Verification items for this drawing (mm, ordinates from the low corner). A direction names the side the tool comes from. Round coordinates to 2 decimals unless told otherwise and drop trailing zeros. Loops run counter-clockwise (first coordinate to the right, second up) from the corner with the lowest first, then second, coordinate; pieces in that order, holes last. Notation, with made-up numbers: M -3.75,-0.5 L 14.25,-0.5 A16 ccw 14.25,22.5 Z; hole C 2.5,68.5 d3. An arc over 180 degrees is marked long. Answer as CSV lines item,"result".
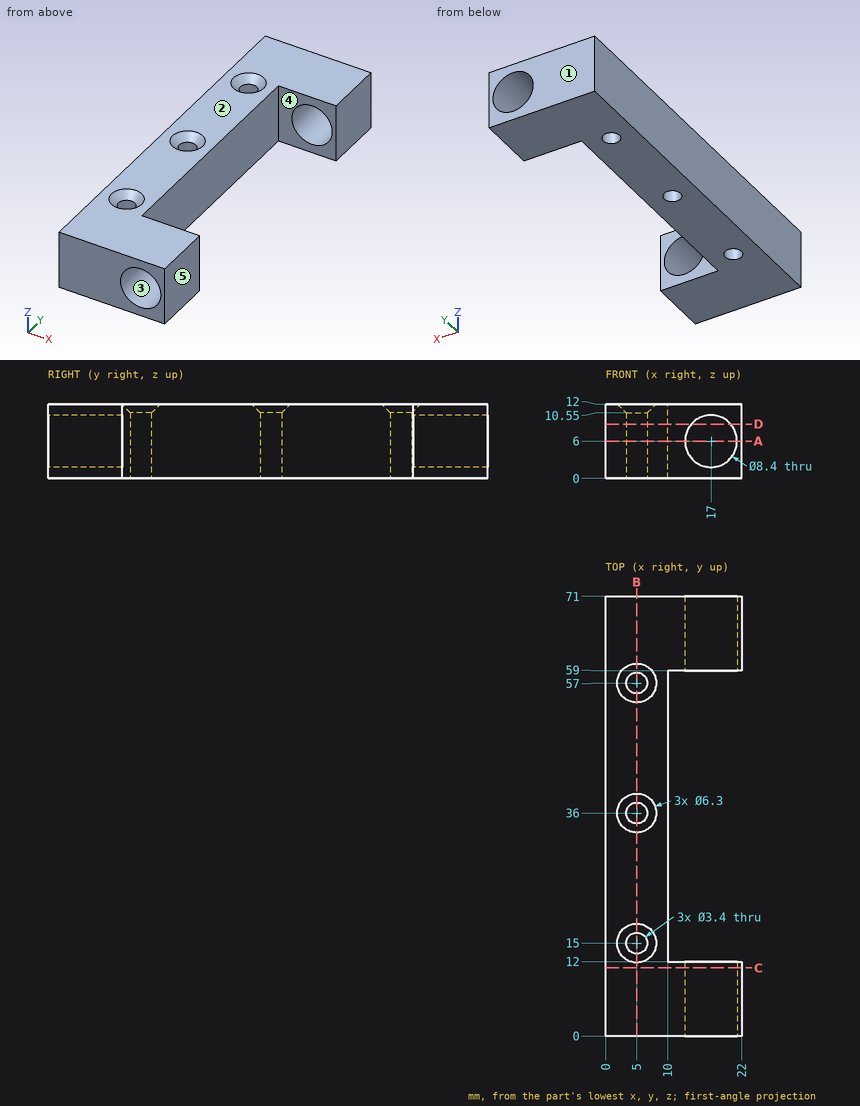
1) Section check C-C (y = 11). Record the cut outline in (x, z), plus the area to 3 significant figures.
Here are the results:
outline,"M 0,0 L 22,0 L 22,12 L 0,12 Z; hole C 17,6 d8.4"
area,"209 mm^2"
2) Section check D-D (z = 8.75). Record the cut outline in (x, y), plus the area to 3 significant figures.
Here are the results:
outline,"M 0,0 L 13.83,0 L 13.83,12 L 10,12 L 10,59 L 13.83,59 L 13.83,71 L 0,71 Z; M 20.17,0 L 22,0 L 22,12 L 20.17,12 Z; M 20.17,59 L 22,59 L 22,71 L 20.17,71 Z; hole C 5,15 d3.4; hole C 5,36 d3.4; hole C 5,57 d3.4"
area,"818 mm^2"
3) Draft check along Z on the marked faces 1, 2 and 3. Enter one of: +Z half, -Z half, draft (parallel to the pull), parting line (faces both ways), or undercut.
Here are the results:
face 1,"draft"
face 2,"+Z half"
face 3,"undercut"
4) Section check B-B (x = 5). Record the cut outline in (y, z), plus the area to 3 significant figures.
Here are the results:
outline,"M 0,0 L 13.3,0 L 13.3,10.55 L 11.85,12 L 0,12 Z; M 16.7,0 L 34.3,0 L 34.3,10.55 L 32.85,12 L 18.15,12 L 16.7,10.55 Z; M 37.7,0 L 55.3,0 L 55.3,10.55 L 53.85,12 L 39.15,12 L 37.7,10.55 Z; M 58.7,0 L 71,0 L 71,12 L 60.15,12 L 58.7,10.55 Z"
area,"723 mm^2"
5) Section check A-A (z = 6). Record the cut outline in (x, y).
Here are the results:
outline,"M 0,0 L 12.8,0 L 12.8,12 L 10,12 L 10,59 L 12.8,59 L 12.8,71 L 0,71 Z; M 21.2,0 L 22,0 L 22,12 L 21.2,12 Z; M 21.2,59 L 22,59 L 22,71 L 21.2,71 Z; hole C 5,15 d3.4; hole C 5,36 d3.4; hole C 5,57 d3.4"
6) Set-up check for the marked faces 4 and 5: record each of +Z, -Z, +X, -X, +Y, -Y from which the full face is reachable in a straight line by a thin tool's end or side.
Here are the results:
face 4,"+Z, -Z, +X"
face 5,"+Z, -Z, +X, +Y, -Y"
7) Go/stop test with flat-tipped pins: pin 1 (6 mm diameter, centred on y = 36.5, z = 5, fed in from +X); pin 2 (2.5 mm diameter, centred on x = 5, y = 15, fed in from -Z); pin 3 (4.5 mm diameter, centred on x = 5, y = 57, fed in from +Z). Record where each tip stops, or that it passes through.
Here are the results:
pin 1,"stops at x = 10"
pin 2,"passes through"
pin 3,"stops at z = 11.1"
8) Material ranges on probe 1 along Y at (x, z) = (5, 8.5); probe 2 along X at (y, z) = (15, 7.75); probe 3 along X at (y, z) = (4.5, 6.25), recorded low to high.
Here are the results:
probe 1,"y = 0 to 13.3, 16.7 to 34.3, 37.7 to 55.3, 58.7 to 71"
probe 2,"x = 0 to 3.3, 6.7 to 10"
probe 3,"x = 0 to 12.81, 21.19 to 22"
